Verification items for the finished model (mm, model axes). Face numbers are marked on the shaded views. A direction names the side the tool comes from. Coordinates: 2 decimals unless noted, no trailing zeros. Write each loop counter-clockwise with the first axis right and the second up, starting at its lowest first coordinate (ties: lowest second). Pieces come first, ordered by that corner, then holes. Notation, with made-up numbers: (-10, -0.75) -> (20, -0.75) arc R23 ccw to (20, 30.25) -> close; hole circle Ø3 at (-28, 84). An arc over 180 degrees is marked (long way). Answer in a Markdown table with one row per item.
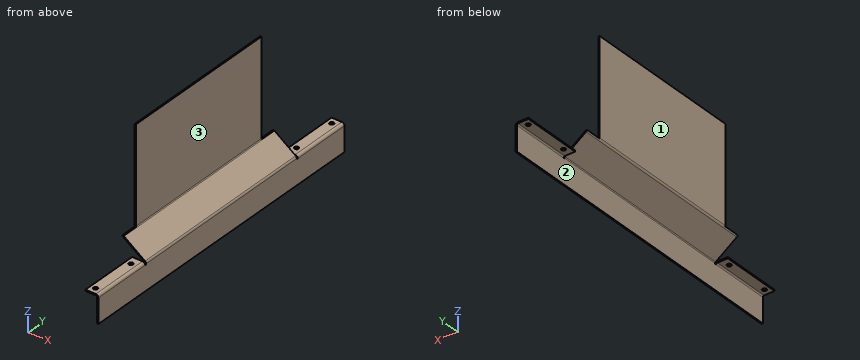
```python
from build123d import *

# Parameters (mm, degrees)
F1_DEPTH  = 150
F3_DEPTH  = 95
F4_W      = 2
F4_H      = 56
F6_DEPTH  = 25
F5_W      = 55.4491758279
F5_H      = 188.3780552482
F7_DEPTH  = 50
F8_R      = 2
F9_R      = 4
F10_R     = 3.25
F11_DEPTH = 25


# Not quite as in the source:
# - a pattern or mirror of a feature is missing from the dataset's text; its kind, count and spacing are read off the source's solid


with BuildPart() as f1:
    # F0 (on Front) → F1 (new body, symmetric)
    with BuildSketch(Plane.XZ):
        Polygon((1, -26), (1, -66), (3, -66), (3, -24.9707642094), (-32, 0.0292357906), (-32, 149), (-34, 149), (-34, -1), align=None)
    extrude(amount=F1_DEPTH, both=True)

    # F2 (on face) → F3 (join)
    with BuildSketch(Plane.XZ.offset(150)):
        Polygon((1.6409301068, -24), (3, -24.9707642094), (3, -24), align=None)
        Polygon((-17, -26), (1, -26), (-1.8, -24), (-17, -24), align=None)
        Polygon((1, -27.0292357906), (1, -66), (3, -66), (3, -24.9707642094), (1.6409301068, -24), (-1.8, -24), (1, -26), align=None)
    f3 = extrude(amount=F3_DEPTH)

    # F3_copies: F3 across plane
    add(f3.mirror(Plane.ZX))

    # F4 (on face) → F6 (cut)
    with BuildSketch(Plane.YZ.offset(3)):
        with Locations((-151, 0)):
            Rectangle(F4_W, F4_H)
        with Locations((151, 0)):
            Rectangle(F4_W, F4_H)
    extrude(amount=-F6_DEPTH, mode=Mode.SUBTRACT)

    # F5 (on face) → F7 (cut)
    with BuildSketch(Plane.YZ.offset(3)):
        with Locations((152.724587914, 94.1890276241)):
            Rectangle(F5_W, F5_H)
        with Locations((-152.724587914, 94.1890276241)):
            Rectangle(F5_W, F5_H)
    extrude(amount=-F7_DEPTH, mode=Mode.SUBTRACT)

    # F8
    f8_edges = [f1.edges().sort_by_distance(p)[0] for p in [
        (-32, 0, 0.029236),
        (1, -198.5, -26),
        (1, 0, -26),
        (1, 198.5, -26),
    ]]
    fillet(f8_edges, radius=F8_R)

    # F9
    f9_edges = [f1.edges().sort_by_distance(p)[0] for p in [
        (3, -198.5, -24),
        (3, 0, -24.970764),
        (-34, 0, -1),
        (3, 198.5, -24),
    ]]
    fillet(f9_edges, radius=F9_R)

    # F10 (on face) → F11 (cut)
    with BuildSketch(Plane.XY.offset(-24)):
        with Locations((-9, 235)):
            Circle(F10_R)
        with Locations((-9, 165)):
            Circle(F10_R)
        with Locations((-9, -165)):
            Circle(F10_R)
        with Locations((-9, -235)):
            Circle(F10_R)
    extrude(amount=-F11_DEPTH, mode=Mode.SUBTRACT)


solid = f1.part
```
1. Material ranges on probe 1 along Y at (x, z) = (-9, -25); probe 2 along X at (y, z) = (165, -24.7); probe 3 along X at (y, z) = (112, 137), recorded low to high. Write a range as from..to.
Findings below:
| item | result |
|---|---|
| probe 1 | y = -245..-238.25, -231.75..-168.25, -161.75..-152, 152..161.75, 168.25..231.75, 238.25..245 |
| probe 2 | x = -17..-12.25, -5.75..1.26 |
| probe 3 | x = -34..-32 |
2. Sectioned sample at C-C, the plane y = -145.5. Record the cut outline in (x, z).
Findings below:
| item | result |
|---|---|
| outline | (-33.86, 0) arc R4 ccw to (-32.32, -2.2) -> (0.16, -25.4) arc R2 cw to (1, -27.03) -> (1, -66) -> (3, -66) -> (3, -27.03) arc R4 ccw to (1.32, -23.77) -> (-31.16, -0.57) arc R2 cw to (-31.7, 0) -> close |
3. Sectioned sample at A-A, the plane y = -23.5. Record the cut outline in (x, z).
Findings below:
| item | result |
|---|---|
| outline | (-34, 1.06) arc R4 ccw to (-32.32, -2.2) -> (0.16, -25.4) arc R2 cw to (1, -27.03) -> (1, -66) -> (3, -66) -> (3, -27.03) arc R4 ccw to (1.32, -23.77) -> (-31.16, -0.57) arc R2 cw to (-32, 1.06) -> (-32, 149) -> (-34, 149) -> close |
4. Sectioned sample at B-B, the plane z = 129.5. Record the cut outline in (x, y).
Findings below:
| item | result |
|---|---|
| outline | (-34, -125) -> (-32, -125) -> (-32, 125) -> (-34, 125) -> close |
5. Access from +Z, -Z, +X, -X, +Y, -Y to the whole of each face (thin tool, end or side, straight path). Record for the marked faces 1, 2 and 3.
Findings below:
| item | result |
|---|---|
| face 1 | +Z, -Z, -X, +Y, -Y |
| face 2 | -Z, -X, +Y, -Y |
| face 3 | +Z, +X, +Y, -Y |
6. Go/stop test with flat-tipped pins: pin 1 (17.5 mm diameter, centred on x = -7, y = 216, fed in from +Z); pin 2 (1.2 mm diameter, centred on x = -32.5, z = 102, fed in from -Y); pin 3 (12 mm diameter, centred on y = 86, z = 18.5, fed in from +X); pin 4 (4 mm diameter, centred on x = -16.5, z = -20.5, fed in from +Y) (3 decimals). Record where each tip stops, or that it passes through.
Findings below:
| item | result |
|---|---|
| pin 1 | stops at z = -24 |
| pin 2 | stops at y = -125 |
| pin 3 | stops at x = -32 |
| pin 4 | passes through |
7. Sectioned sample at D-D, the plane x = -26.5. Record the cut outline in (y, z).
Findings below:
| item | result |
|---|---|
| outline | (-150, -6.36) -> (150, -6.36) -> (150, -3.9) -> (-150, -3.9) -> close |
